Source: three-view drawing plus pictorial views. Frame: mm from the lowest corner of the part. A direction names the side the tool comes from. Round coordinates to 2 decimals unless told otherwise and drop trailing zeros. Order: outer loops, then holes, each group sorted by start corner. A loop starts at its lowest first (then second) coordinate and runs counter-clockwise, first axis right, second up. Notation, with made-up numbers: (-6.75, 19) -> (-2.75, 19) arc R15 cw to (-2.75, 25) -> close; hole circle Ø8 at (1, 20.25). An arc over 180 degrees is marked (long way). Answer as CSV lines item,"result". Start each with the question number.
1) Mould query, pull axis Y, two halves, no side actions, for the marked faces 1, 2 and 3. Classes: +Y half, -Y half, draft (parallel to the pull), parting line (faces both ways), or undercut.
2) Line query: L1, parallel to Z at x = 40, y = 50.5; L2, parallel to Y at x = 117, z = 76; L3, parallel to X at y = 61, z = 82.5. Output: solid intervals per line, ascending.
3) Section query B-B, the plane x = 116. Output: boundary loops of the cut face in (y, z) (1 decimal), and give its area (3 significant figures).
4) Section query A-A, the plane z = 86. Output: boundary loops of the cut face in (x, y).
5) Access query for the marked faces 4, 5, 6 and 7. Directions: +Z, -Z, +X, -X, +Y, -Y. A direction counts if a zero-diameter tool reaches every point of the face in a straight line with its end or side. Return the directions, or none.
6) First-contact query: P1, Ø2, axis at x = 67, y = 29, coming from the +Z side; P2, Ø4.5, axis at x = 116, y = 10, coming from the -Z side; P3, Ø2, axis at y = 60, z = 11, coming from the -X side. Flat tips, straight axial feed; report the tip coordinate or a pass-through.
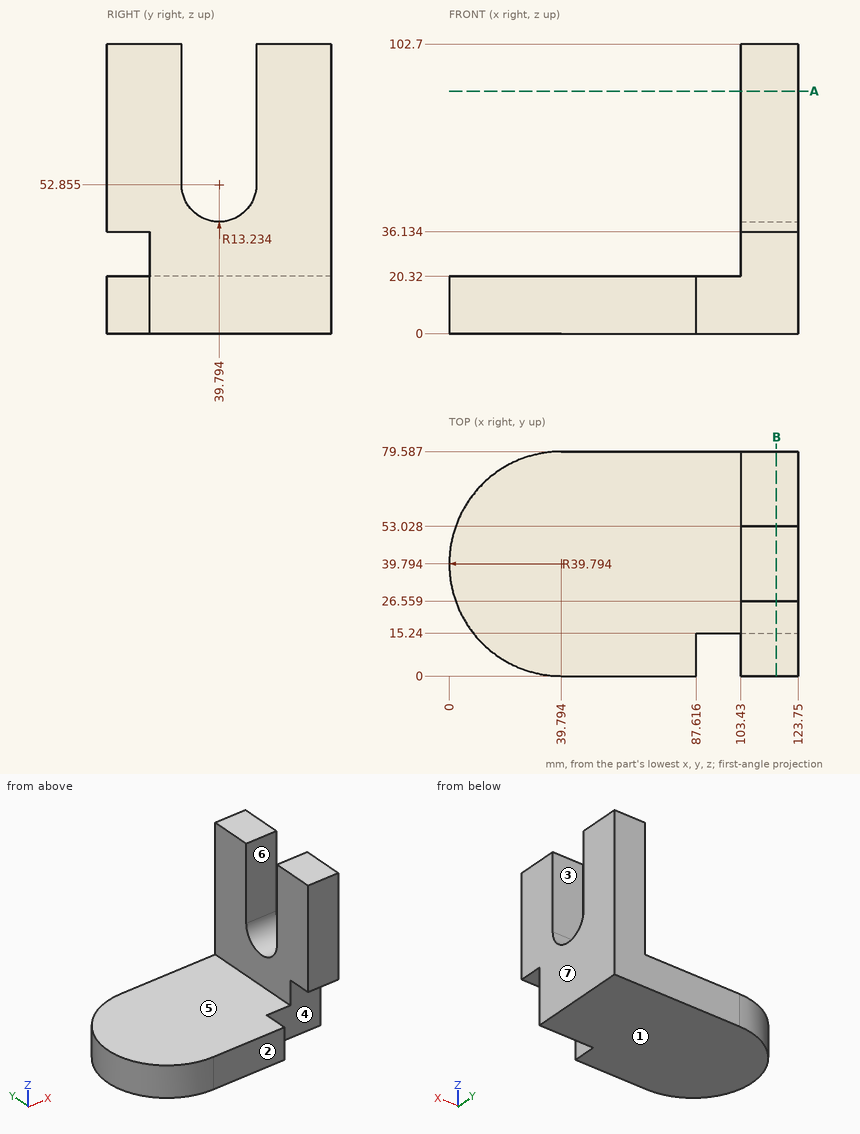
Findings:
1,face 1,"draft"
1,face 2,"-Y half"
1,face 3,"undercut"
2,L1,"z = 0 to 20.32"
2,L2,"y = 0 to 26.56, 53.03 to 79.59"
2,L3,"x = 103.43 to 123.75"
3,outline,"(0, 36.1) -> (15.2, 36.1) -> (15.2, 0) -> (79.6, 0) -> (79.6, 102.7) -> (53, 102.7) -> (53, 52.9) arc R13.2 cw to (26.6, 52.9) -> (26.6, 102.7) -> (0, 102.7) -> close"
3,area,"6,030 mm^2"
4,outline,"(103.43, 0) -> (123.75, 0) -> (123.75, 26.56) -> (103.43, 26.56) -> close; (103.43, 53.03) -> (123.75, 53.03) -> (123.75, 79.59) -> (103.43, 79.59) -> close"
5,face 4,"-Z, +X, -Y"
5,face 5,"+Z, -X, +Y, -Y"
5,face 6,"+Z, +X, -X"
5,face 7,"+Z, -Z, +X, +Y, -Y"
6,P1,"stops at z = 20.32"
6,P2,"stops at z = 36.13"
6,P3,"stops at x = 4.94"
